```python
from build123d import *
from build123d.topology import SkipClean

# Parameters (mm, degrees)
SKETCH1_R                = 2.25
BOSS_EXTRUDE1_DEPTH      = 2
SKETCH2_R                = 15
BOSS_EXTRUDE2_DEPTH      = 9
BOSS_EXTRUDE3_DEPTH      = 5
SKETCH4_R                = 1.5
BOSS_EXTRUDE4_DEPTH      = 2
FILLET1_R                = 3
BOSS_EXTRUDE5_DEPTH      = 8
BOSS_EXTRUDE5_DEPTH_BACK = 8
SKETCH5_R                = 22.5
FILLET2_R                = 3
SKETCH6_R                = 1.5
BOSS_EXTRUDE6_DEPTH      = 25


with BuildPart() as part:
    # Sketch1 → Boss-Extrude1 (new body)
    with BuildSketch(Plane(origin=(0, 0, 0), x_dir=(1, 0, 0), z_dir=(0, 1, 0))):
        with BuildLine():
            Line((-19, 21), (19, 21))
            ThreePointArc((19, 21), (20.414213562, 20.414213562), (21, 19))
            Line((21, 19), (21, -19))
            ThreePointArc((21, -19), (20.414213562, -20.414213562), (19, -21))
            Line((19, -21), (-19, -21))
            ThreePointArc((-19, -21), (-20.414213562, -20.414213562), (-21, -19))
            Line((-21, -19), (-21, 19))
            ThreePointArc((-21, 19), (-20.414213562, 20.414213562), (-19, 21))
        make_face()
        with Locations(Location((-15, 15, 0), (0, 0, 270))):
            Circle(SKETCH1_R, mode=Mode.SUBTRACT)
        with Locations(Location((15, 15, 0), (0, 0, 90))):
            Circle(SKETCH1_R, mode=Mode.SUBTRACT)
        with Locations(Location((15, -15, 0), (0, 0, 270))):
            Circle(SKETCH1_R, mode=Mode.SUBTRACT)
        with Locations(Location((-15, -15, 0), (0, 0, 90))):
            Circle(SKETCH1_R, mode=Mode.SUBTRACT)
    extrude(amount=BOSS_EXTRUDE1_DEPTH)

    # Sketch2 → Boss-Extrude2 (add)
    with BuildSketch(Plane(origin=(0, 2, 0), x_dir=(1, 0, 0), z_dir=(0, 1, 0))):
        with Locations(Location((0, 0, 0), (0, 0, 270))):
            Circle(SKETCH2_R)
    extrude(amount=BOSS_EXTRUDE2_DEPTH)

    # Sketch3 → Boss-Extrude3 (add)
    with SkipClean():  # the faces are left unmerged after this step: merging them gives an invalid solid
        with BuildSketch(Plane(origin=(0, 11, 0), x_dir=(1, 0, 0), z_dir=(0, 1, 0))):
            with BuildLine():
                Line((-25, 12.5), (-8.291561976, 12.5))
                ThreePointArc((-8.291561976, 12.5), (15, 0), (-8.291561976, -12.5))
                Line((-8.291561976, -12.5), (-25, -12.5))
                Line((-25, -12.5), (-25, 12.5))
            make_face()
        extrude(amount=BOSS_EXTRUDE3_DEPTH)

    # Sketch4 → Boss-Extrude4 (add)
    with SkipClean():  # the faces are left unmerged after this step: merging them gives an invalid solid
        with BuildSketch(Plane.XY.offset(12.5)):
            with BuildLine():
                Line((-25, 16), (-26.988009316, 44.653931998))
                ThreePointArc((-26.988009316, 44.653931998), (-23.614360312, 49.732213096), (-17.840451563, 47.774555244))
                Line((-17.840451563, 47.774555244), (3.354219012, 16))
                Line((3.354219012, 16), (-25, 16))
            make_face()
            with Locations((-22, 45)):
                Circle(SKETCH4_R, mode=Mode.SUBTRACT)
        boss_extrude4 = extrude(amount=-BOSS_EXTRUDE4_DEPTH)

    # Mirror1: Boss-Extrude4 across plane
    with SkipClean():  # the faces are left unmerged after this step: merging them gives an invalid solid
        add(boss_extrude4.mirror(Plane.XY))

    # Fillet1
    # the kernel refuses this fillet: 3 mm, written as the material it adds along each edge
    with BuildSketch(Plane(origin=(10.854219012, 16, 12.5), x_dir=(0, 0, 1), z_dir=(-1, 0, 0))) as fillet1_piece_1_section:
        with BuildLine():
            CenterArc((FILLET1_R, FILLET1_R), FILLET1_R, 180, 90)
            Line((0, FILLET1_R), (0, 0))
            Line((0, 0), (FILLET1_R, 0))
        make_face()
    fillet1_piece_1 = extrude(amount=26.645780988, mode=Mode.PRIVATE)
    fillet1_piece_1 = fillet1_piece_1 & Plane(origin=(0, 16.711249506, 0), x_dir=(-0.5527707983925666, 0, -0.8333333333333335), z_dir=(0, -1, 0)) * Cylinder(15, 66, mode=Mode.PRIVATE)
    fillet1_piece_1 = split(fillet1_piece_1, bisect_by=Plane(origin=(1.321328689, 19.047661706, 13.078964715), z_dir=(-0.8319096874112317, -0.5549110487198348, 0)), keep=Keep.TOP, mode=Mode.PRIVATE)
    add(fillet1_piece_1)
    with BuildSketch(Plane(origin=(10.854219012, 16, -12.5), x_dir=(0, 0, -1), z_dir=(-1, 0, 0))) as fillet1_piece_2_section:
        with BuildLine():
            CenterArc((FILLET1_R, -FILLET1_R), FILLET1_R, 90, 90)
            Line((0, -FILLET1_R), (0, 0))
            Line((0, 0), (FILLET1_R, 0))
        make_face()
    fillet1_piece_2 = extrude(amount=26.645780988, mode=Mode.PRIVATE)
    fillet1_piece_2 = fillet1_piece_2 & Plane(origin=(0, 16.711251501, 0), x_dir=(-0.5527707983925666, 0, -0.8333333333333335), z_dir=(0, -1, 0)) * Cylinder(15, 66, mode=Mode.PRIVATE)
    fillet1_piece_2 = split(fillet1_piece_2, bisect_by=Plane(origin=(1.321327042, 19.047664174, -13.078969709), z_dir=(-0.8319096874112317, -0.5549110487198348, 0)), keep=Keep.TOP, mode=Mode.PRIVATE)
    add(fillet1_piece_2)



with BuildPart() as body_2:
    # Sketch5 → Boss-Extrude5 (new, two sides: drawn at the far end of the back side and taken through both)
    with BuildSketch(Plane.XY.offset(-BOSS_EXTRUDE5_DEPTH_BACK)):
        with Locations((-22, 45)):
            Circle(SKETCH5_R)
    extrude(amount=BOSS_EXTRUDE5_DEPTH + BOSS_EXTRUDE5_DEPTH_BACK)

    # Fillet2
    fillet2_edges = [body_2.edges().sort_by_distance(p)[0] for p in [
        (-44.5, 45, 8),
        (-44.5, 45, -8),
    ]]
    fillet(fillet2_edges, radius=FILLET2_R)


with BuildPart() as part_1:
    add(part.part)

    add(body_2.part)  # Boss-Extrude6 merges body 2
    # Sketch6 → Boss-Extrude6 (add)
    with BuildSketch(Plane.XY.offset(12.5)):
        with Locations((-22, 45)):
            Circle(SKETCH6_R)
    extrude(amount=-BOSS_EXTRUDE6_DEPTH)


solid = part_1.part
```
Geometry check sheet. Reference: the model listing, model coordinates, mm. A direction names the side the tool comes from. Round coordinates to 2 decimals unless told otherwise and drop trailing zeros. Write each loop counter-clockwise with the first axis right and the second up, starting at its lowest first coordinate (ties: lowest second). Pieces come first, ordered by that corner, then holes. Notation, with made-up numbers: (11, -13) - (28, -13) arc R17 ccw to (28, 14) - close; hole circle Ø6 at (18.5, 83.25). An arc over 180 degrees is marked (long way). Write each question's results on one line, items separated by ' | '.
(1) Sectioned sample at C-C, the plane y = 12.5. Enter the section's corners in (x, z).
Computed:
outline: (-25, -12.5) - (-8.29, -12.5) arc R15 ccw (long way) to (-8.29, 12.5) - (-25, 12.5) - close
(2) Set-up check for faces 1 (the face through (-22.325, 43.536, 9.268)), 2 (the face through (21, 1, 0)), 3 (the face through (-21, 1, 0)), 4 (the face through (-16, 31, 12.5)), 5 (the face through (-25.98, 30.13, 11.51)): record each of +Z, -Z, +X, -X, +Y, -Y from which the full face is reachable in a straight line by a thin tool's end or side.
Computed:
face 1: none | face 2: +Z, -Z, +X, +Y, -Y | face 3: +Z, -Z, -X, -Y | face 4: +Z, -X, +Y | face 5: +Z, -X, -Y
(3) Draft check along Z on faces 6 (the face through (-25.98, 30.13, -11.51)), 7 (the face through (-22.325, 43.536, -9.233)), 8 (the face through (-20.4, 0.99, 20.43)). Enter one of: pulls with the +Z half, pulls with the -Z half, needs draft (parallel to the pull), parting line crosses it, or undercut.
Computed:
face 6: needs draft | face 7: undercut | face 8: pulls with the +Z half
(4) Sectioned sample at D-D, the plane z = 6.5. Enter the section's corners in (x, y), plus the area to 3 significant figures.
Computed:
outline: circle Ø44.2 at (-22, 45); (-25, 11) - (-13.52, 11) - (-13.52, 2) - (-21, 2) - (-21, 0) - (21, 0) - (21, 2) - (13.52, 2) - (13.52, 16) - (-25, 16) - close | area: 2,050 mm^2
(5) Sectioned sample at A-A, the plane z = 0. Enter the section's corners in (x, y).
Computed:
outline: circle Ø45 at (-22, 45); (-25, 11) - (-15, 11) - (-15, 2) - (-21, 2) - (-21, 0) - (21, 0) - (21, 2) - (15, 2) - (15, 16) - (-25, 16) - close
(6) Depth check by flat-ended pin: pin 1 Ø8 at (y, z) = (47.5, -4.5) entering from +X; pin 2 Ø1.5 at (y, z) = (46, -9) entering from +X; pin 3 Ø6 at (x, z) = (12, -16.5) entering from +Y; pin 4 Ø8 at (y, z) = (49, -1.5) entering from -X. Enter the tip coordinate at first touch or a pass-through.
Computed:
pin 1: stops at x = 0.5 | pin 2: stops at x = -20.52 | pin 3: stops at y = 2 | pin 4: stops at x = -44.5
(7) Thickness scan on probe 1 along X at (y, z) = (0.6, 15); probe 2 along Y at (x, z) = (-17, 6.5); probe 3 along Y at (x, z) = (-17, 19). Record the ranges inside material, lowest first. Write a range as from..to.
Computed:
probe 1: x = -21..-17.25, -12.75..12.75, 17.25..21 | probe 2: y = 0..2, 11..16, 23.48..66.52 | probe 3: y = 0..2
(8) Sectioned sample at B-B, the plane x = -22. Enter the section's corners in (y, z), plus the area to 3 significant figures.
Computed:
outline: (11, -12.5) - (50, -12.5) - (50, -10.5) - (46.5, -10.5) - (46.5, -8) - (64.5, -8) arc R3 ccw to (67.5, -5) - (67.5, 5) arc R3 ccw to (64.5, 8) - (46.5, 8) - (46.5, 10.5) - (50, 10.5) - (50, 12.5) - (11, 12.5) - close; hole (16, -10.5) - (43.5, -10.5) - (43.5, -8) - (25.5, -8) arc R3 cw to (22.5, -5) - (22.5, 5) arc R3 cw to (25.5, 8) - (43.5, 8) - (43.5, 10.5) - (16, 10.5) - close | area: 988 mm^2
